```python
from build123d import *
from OCP.BRepFilletAPI import BRepFilletAPI_MakeChamfer

# Parameters (mm, degrees)
SKETCH1_W           = 76.962
SKETCH1_H           = 46.99
BOSS_EXTRUDE1_DEPTH = 20.066
SKETCH2_W           = 72.68972
SKETCH2_H           = 42.7482
CUT_EXTRUDE1_DEPTH  = 2.54
SKETCH3_W           = 69.38772
SKETCH3_H           = 39.37
CUT_EXTRUDE2_DEPTH  = 16.256
CHAMFER1_SIZE       = 2.54
SKETCH6_R           = 1.5875
BOSS_EXTRUDE2_DEPTH = 2.54
CUT_EXTRUDE5_DEPTH  = 97.402641646
FILLET1_R           = 2.54
SKETCH9_R           = 1.5875
BOSS_EXTRUDE3_DEPTH = 2.54
SKETCH12_W          = 1.27
SKETCH12_H          = 2.54
BOSS_EXTRUDE5_DEPTH = 1.27
CHAMFER4_SIZE       = 2.54
CHAMFER4_SIZE_2     = 9.479409052
SKETCH13_W          = 6.35
SKETCH13_H          = 11.176
SKETCH13_W_2        = 13.97
SKETCH13_H_2        = 6.35
CUT_EXTRUDE7_DEPTH  = 104.876082503
SKETCH14_W          = 2.54
SKETCH14_H          = 1.27
BOSS_EXTRUDE6_DEPTH = 2.54
CHAMFER5_SIZE       = 2.54000495
CHAMFER5_SIZE_2     = 9.479427523
CHAMFER6_SIZE       = 2.54


with BuildPart() as part:
    # Sketch1 → Boss-Extrude1 (new body)
    with BuildSketch(Plane(origin=(0, 0, 0), x_dir=(1, 0, 0), z_dir=(0, 1, 0))):
        with Locations((38.481, 23.495)):
            Rectangle(SKETCH1_W, SKETCH1_H)
    extrude(amount=BOSS_EXTRUDE1_DEPTH)

    # Sketch2 → Cut-Extrude1 (cut)
    with BuildSketch(Plane(origin=(0, 20.066, 0), x_dir=(1, 0, 0), z_dir=(0, 1, 0))):
        with Locations((38.481, 23.495)):
            Rectangle(SKETCH2_W, SKETCH2_H)
    extrude(amount=-CUT_EXTRUDE1_DEPTH, mode=Mode.SUBTRACT)

    # Sketch3 → Cut-Extrude2 (cut)
    with BuildSketch(Plane(origin=(0, 17.526, 0), x_dir=(1, 0, 0), z_dir=(0, 1, 0))):
        with Locations((38.481, 23.495)):
            Rectangle(SKETCH3_W, SKETCH3_H)
    extrude(amount=-CUT_EXTRUDE2_DEPTH, mode=Mode.SUBTRACT)

    # Chamfer1
    chamfer1_edges = [part.edges().sort_by_distance(p)[0] for p in [
        (0, 10.033, -46.99),
        (76.962, 10.033, -46.99),
        (76.962, 10.033, 0),
        (0, 10.033, 0),
    ]]
    chamfer(chamfer1_edges, length=CHAMFER1_SIZE)

    # Sketch6 → Boss-Extrude2 (add)
    # profile 1 of 4: a face of its own
    with BuildSketch(Plane.XZ):
        with BuildLine():
            Line((3.4925, 3.81), (3.4925, 0))
            Line((3.4925, 0), (11.7475, 0))
            Line((11.7475, 0), (11.7475, 3.81))
            ThreePointArc((11.7475, 3.81), (7.62, 7.9375), (3.4925, 3.81))
        make_face()
        with Locations(Location((7.62, 3.81, 0), (0, 0, 270))):
            Circle(SKETCH6_R, mode=Mode.SUBTRACT)
    # profile 2 of 4: a face of its own
    with BuildSketch(Plane.XZ):
        with BuildLine():
            Line((11.7475, -46.99), (11.7475, -50.8))
            ThreePointArc((11.7475, -50.8), (7.62, -54.9275), (3.4925, -50.8))
            Line((3.4925, -50.8), (3.4925, -46.99))
            Line((3.4925, -46.99), (11.7475, -46.99))
        make_face()
        with Locations(Location((7.62, -50.8, 0), (0, 0, 90))):
            Circle(SKETCH6_R, mode=Mode.SUBTRACT)
    # profile 3 of 4: a face of its own
    with BuildSketch(Plane.XZ):
        with BuildLine():
            Line((73.4695, -50.8), (73.4695, -46.99))
            Line((73.4695, -46.99), (65.2145, -46.99))
            Line((65.2145, -46.99), (65.2145, -50.8))
            ThreePointArc((65.2145, -50.8), (69.342, -54.9275), (73.4695, -50.8))
        make_face()
        with Locations(Location((69.342, -50.8, 0), (0, 0, 270))):
            Circle(SKETCH6_R, mode=Mode.SUBTRACT)
    # profile 4 of 4: a face of its own
    with BuildSketch(Plane.XZ):
        with BuildLine():
            Line((65.2145, 0), (65.2145, 3.81))
            ThreePointArc((65.2145, 3.81), (69.342, 7.9375), (73.4695, 3.81))
            Line((73.4695, 3.81), (73.4695, 0))
            Line((73.4695, 0), (65.2145, 0))
        make_face()
        with Locations(Location((69.342, 3.81, 0), (0, 0, 90))):
            Circle(SKETCH6_R, mode=Mode.SUBTRACT)
    extrude(amount=-BOSS_EXTRUDE2_DEPTH)

    # Sketch7 → Cut-Extrude5 (cut, through all)
    with BuildSketch(Plane(origin=(0, 1.27, 0), x_dir=(1, 0, 0), z_dir=(0, 1, 0))):
        Polygon((15.896309728, 40.64), (61.065690272, 40.64), (38.481, 26.492218855), align=None)
        Polygon((6.32714, 40.64), (6.32714, 6.35), (33.696415136, 23.495), align=None)
        Polygon((15.964259965, 6.392566228), (60.997740035, 6.392566228), (38.481, 20.497781145), align=None)
        Polygon((70.63486, 40.64), (70.63486, 6.35), (43.265584864, 23.495), align=None)
    extrude(amount=-CUT_EXTRUDE5_DEPTH, mode=Mode.SUBTRACT)

    # Fillet1
    fillet1_edges = [part.edges().sort_by_distance(p)[0] for p in [
        (61.065690272, 0.635, -40.64),
        (38.481, 0.635, -26.492218855),
        (15.896309728, 0.635, -40.64),
        (15.964259965, 0.635, -6.392566228),
        (38.481, 0.635, -20.497781145),
        (60.997740035, 0.635, -6.392566228),
        (43.265584864, 0.635, -23.495),
        (70.63486, 0.635, -40.64),
        (70.63486, 0.635, -6.35),
        (33.696415136, 0.635, -23.495),
        (6.32714, 0.635, -6.35),
        (6.32714, 0.635, -40.64),
    ]]
    fillet(fillet1_edges, radius=FILLET1_R)

    # Sketch9 → Boss-Extrude3 (add)
    # profile 1 of 2: a face of its own
    with BuildSketch(Plane(origin=(0, 20.066, 0), x_dir=(1, 0, 0), z_dir=(0, 1, 0))):
        with BuildLine():
            Line((-3.81, 28.575), (0, 28.575))
            Line((0, 28.575), (0, 18.415))
            Line((0, 18.415), (-3.81, 18.415))
            ThreePointArc((-3.81, 18.415), (-8.89, 23.495), (-3.81, 28.575))
        make_face()
        with Locations(Location((-3.81, 23.495, 0), (0, 0, 270))):
            Circle(SKETCH9_R, mode=Mode.SUBTRACT)
    # profile 2 of 2: a face of its own
    with BuildSketch(Plane(origin=(0, 20.066, 0), x_dir=(1, 0, 0), z_dir=(0, 1, 0))):
        with BuildLine():
            Line((76.962, 18.415), (80.772, 18.415))
            ThreePointArc((80.772, 18.415), (85.852, 23.495), (80.772, 28.575))
            Line((80.772, 28.575), (76.962, 28.575))
            Line((76.962, 28.575), (76.962, 18.415))
        make_face()
        with Locations(Location((80.772, 23.495, 0), (0, 0, 90))):
            Circle(SKETCH9_R, mode=Mode.SUBTRACT)
    extrude(amount=-BOSS_EXTRUDE3_DEPTH)

    # Sketch12 → Boss-Extrude5 (add)
    with BuildSketch(Plane(origin=(0, 2.54, 0), x_dir=(1, 0, 0), z_dir=(0, 1, 0))):
        with Locations((4.1275, -1.27)):
            Rectangle(SKETCH12_W, SKETCH12_H)
        with Locations((11.1125, -1.27)):
            Rectangle(SKETCH12_W, SKETCH12_H)
        with Locations((11.1125, 48.26)):
            Rectangle(SKETCH12_W, SKETCH12_H)
        with Locations((4.1275, 48.26)):
            Rectangle(SKETCH12_W, SKETCH12_H)
        with Locations((72.8345, 48.26)):
            Rectangle(SKETCH12_W, SKETCH12_H)
        with Locations((65.8495, 48.26)):
            Rectangle(SKETCH12_W, SKETCH12_H)
        with Locations((65.8495, -1.27)):
            Rectangle(SKETCH12_W, SKETCH12_H)
        with Locations((72.8345, -1.27)):
            Rectangle(SKETCH12_W, SKETCH12_H)
    extrude(amount=BOSS_EXTRUDE5_DEPTH)

    # Chamfer4
    chamfer4_edges_1 = [part.edges().sort_by_distance(p)[0] for p in [
        (4.1275, 3.81, -46.99),
    ]]
    chamfer4_side_1 = [part.faces().sort_by_distance(p)[0] for p in [
        (4.1275, 3.81, -47.0408),
    ]]
    chamfer4_edges_2 = [part.edges().sort_by_distance(p)[0] for p in [
        (11.1125, 3.81, -46.99),
    ]]
    chamfer4_side_2 = [part.faces().sort_by_distance(p)[0] for p in [
        (11.1125, 3.81, -47.0408),
    ]]
    chamfer4_edges_3 = [part.edges().sort_by_distance(p)[0] for p in [
        (65.8495, 3.81, -46.99),
    ]]
    chamfer4_side_3 = [part.faces().sort_by_distance(p)[0] for p in [
        (65.8495, 3.81, -47.0408),
    ]]
    chamfer4_edges_4 = [part.edges().sort_by_distance(p)[0] for p in [
        (72.8345, 3.81, -46.99),
    ]]
    chamfer4_side_4 = [part.faces().sort_by_distance(p)[0] for p in [
        (72.8345, 3.81, -47.0408),
    ]]
    chamfer4_edges_5 = [part.edges().sort_by_distance(p)[0] for p in [
        (65.8495, 3.81, 0),
    ]]
    chamfer4_side_5 = [part.faces().sort_by_distance(p)[0] for p in [
        (65.8495, 3.81, 0.0508),
    ]]
    chamfer4_edges_6 = [part.edges().sort_by_distance(p)[0] for p in [
        (72.8345, 3.81, 0),
    ]]
    chamfer4_side_6 = [part.faces().sort_by_distance(p)[0] for p in [
        (72.8345, 3.81, 0.0508),
    ]]
    chamfer4_edges_7 = [part.edges().sort_by_distance(p)[0] for p in [
        (11.1125, 3.81, 0),
    ]]
    chamfer4_side_7 = [part.faces().sort_by_distance(p)[0] for p in [
        (11.1125, 3.81, 0.0508),
    ]]
    chamfer4_edges_8 = [part.edges().sort_by_distance(p)[0] for p in [
        (4.1275, 3.81, 0),
    ]]
    chamfer4_side_8 = [part.faces().sort_by_distance(p)[0] for p in [
        (4.1275, 3.81, 0.0508),
    ]]
    chamfer4 = BRepFilletAPI_MakeChamfer(part.part.solid().wrapped)
    for e in chamfer4_edges_1:
        chamfer4.Add(CHAMFER4_SIZE - 0.0001, CHAMFER4_SIZE_2 - 0.0001, e.wrapped, chamfer4_side_1[0].wrapped)
    for e in chamfer4_edges_2:
        chamfer4.Add(CHAMFER4_SIZE - 0.0001, CHAMFER4_SIZE_2 - 0.0001, e.wrapped, chamfer4_side_2[0].wrapped)
    for e in chamfer4_edges_3:
        chamfer4.Add(CHAMFER4_SIZE - 0.0001, CHAMFER4_SIZE_2 - 0.0001, e.wrapped, chamfer4_side_3[0].wrapped)
    for e in chamfer4_edges_4:
        chamfer4.Add(CHAMFER4_SIZE - 0.0001, CHAMFER4_SIZE_2 - 0.0001, e.wrapped, chamfer4_side_4[0].wrapped)
    for e in chamfer4_edges_5:
        chamfer4.Add(CHAMFER4_SIZE - 0.0001, CHAMFER4_SIZE_2 - 0.0001, e.wrapped, chamfer4_side_5[0].wrapped)
    for e in chamfer4_edges_6:
        chamfer4.Add(CHAMFER4_SIZE - 0.0001, CHAMFER4_SIZE_2 - 0.0001, e.wrapped, chamfer4_side_6[0].wrapped)
    for e in chamfer4_edges_7:
        chamfer4.Add(CHAMFER4_SIZE - 0.0001, CHAMFER4_SIZE_2 - 0.0001, e.wrapped, chamfer4_side_7[0].wrapped)
    for e in chamfer4_edges_8:
        chamfer4.Add(CHAMFER4_SIZE - 0.0001, CHAMFER4_SIZE_2 - 0.0001, e.wrapped, chamfer4_side_8[0].wrapped)
    add(Compound.cast(chamfer4.Shape()), mode=Mode.REPLACE)  # a hair under: the kernel refuses the full size

    # Sketch13 → Cut-Extrude7 (cut, through all)
    with BuildSketch(Plane.ZY):
        with Locations((-23.495, 6.858)):
            Rectangle(SKETCH13_W, SKETCH13_H)
        with Locations((-36.195, 4.445)):
            Rectangle(SKETCH13_W_2, SKETCH13_H_2)
        with Locations((-10.795, 4.445)):
            Rectangle(SKETCH13_W_2, SKETCH13_H_2)
    extrude(amount=-CUT_EXTRUDE7_DEPTH, mode=Mode.SUBTRACT)

    # Sketch14 → Boss-Extrude6 (add)
    with BuildSketch(Plane.XZ.offset(-17.526)):
        with Locations((-1.27, -19.05)):
            Rectangle(SKETCH14_W, SKETCH14_H)
        with Locations((-1.27, -27.94)):
            Rectangle(SKETCH14_W, SKETCH14_H)
        with Locations((78.232, -27.94)):
            Rectangle(SKETCH14_W, SKETCH14_H)
        with Locations((78.232, -19.05)):
            Rectangle(SKETCH14_W, SKETCH14_H)
    extrude(amount=BOSS_EXTRUDE6_DEPTH)

    # Chamfer5
    chamfer5_edges_1 = [part.edges().sort_by_distance(p)[0] for p in [
        (76.962, 14.986, -19.05),
    ]]
    chamfer5_side_1 = [part.faces().sort_by_distance(p)[0] for p in [
        (77.012800099, 14.986, -19.05),
    ]]
    chamfer5_edges_2 = [part.edges().sort_by_distance(p)[0] for p in [
        (76.962, 14.986, -27.94),
    ]]
    chamfer5_side_2 = [part.faces().sort_by_distance(p)[0] for p in [
        (77.012800099, 14.986, -27.94),
    ]]
    chamfer5_edges_3 = [part.edges().sort_by_distance(p)[0] for p in [
        (0, 14.986, -27.94),
    ]]
    chamfer5_side_3 = [part.faces().sort_by_distance(p)[0] for p in [
        (-0.050800099, 14.986, -27.94),
    ]]
    chamfer5_edges_4 = [part.edges().sort_by_distance(p)[0] for p in [
        (0, 14.986, -19.05),
    ]]
    chamfer5_side_4 = [part.faces().sort_by_distance(p)[0] for p in [
        (-0.050800099, 14.986, -19.05),
    ]]
    chamfer5 = BRepFilletAPI_MakeChamfer(part.part.solid().wrapped)
    for e in chamfer5_edges_1:
        chamfer5.Add(CHAMFER5_SIZE - 0.0001, CHAMFER5_SIZE_2 - 0.0001, e.wrapped, chamfer5_side_1[0].wrapped)
    for e in chamfer5_edges_2:
        chamfer5.Add(CHAMFER5_SIZE - 0.0001, CHAMFER5_SIZE_2 - 0.0001, e.wrapped, chamfer5_side_2[0].wrapped)
    for e in chamfer5_edges_3:
        chamfer5.Add(CHAMFER5_SIZE - 0.0001, CHAMFER5_SIZE_2 - 0.0001, e.wrapped, chamfer5_side_3[0].wrapped)
    for e in chamfer5_edges_4:
        chamfer5.Add(CHAMFER5_SIZE - 0.0001, CHAMFER5_SIZE_2 - 0.0001, e.wrapped, chamfer5_side_4[0].wrapped)
    add(Compound.cast(chamfer5.Shape()), mode=Mode.REPLACE)  # a hair under: the kernel refuses the full size

    # Chamfer6
    chamfer6_edges = [part.edges().sort_by_distance(p)[0] for p in [
        (75.06843, 7.62, -43.18),
        (1.89357, 7.62, -43.18),
        (75.06843, 7.62, -29.21),
        (1.89357, 7.62, -29.21),
        (75.06843, 7.62, -17.78),
        (1.89357, 7.62, -17.78),
        (75.06843, 7.62, -3.81),
        (1.89357, 7.62, -3.81),
    ]]
    chamfer(chamfer6_edges, length=CHAMFER6_SIZE)


solid = part.part
```
Can you work these out from the model? Positions are in its coordinate system, mm. A direction names the side the tool comes from. Coordinates: 2 decimals unless noted, no trailing zeros. Write each loop counter-clockwise with the first axis right and the second up, starting at its lowest first coordinate (ties: lowest second). Pieces come first, ordered by that corner, then holes. Notation, with made-up numbers: M 28,10 L 35,10 A20 cw 35,44 Z; hole C 37.25,-31 d4. An arc over 180 degrees is marked long. Write item = value, one per line. Start each with the question number.
Q1. If we section it at C-C, the plane z = -1: Write out the boundary of the cut face in (x, y), then the cut area to 3 significant figures.
Q2. If we section it at A-A, the plane x = 7.62: Write out the boundary of the cut face in (y, z).
Q3. I'm going to push flat-ended pins straight in: pin 1 (1.3 mm diameter, centred on x = 77.5, y = 13, fed in from +Z); pin 2 (5 mm diameter, centred on y = 5, z = -4.5, fed in from +X); pin 3 (3 mm diameter, centred on y = 10, z = -48, fed in from -X). Where does each tip first touch, or does it pass through?
Q4. Thinking about a two-plate mould opening in X: for faces 5 (the face through (72.83, 8.62, 1.25)), 6 (the face through (-1.252, 10.18, -19.059)), 7 (the face through (73.175, 13, -23)), which applies, released by +X, released by -X, zero draft, split by the parting line, or undercut?
Q5. On a 3-axis mill with a long thin cutter (end or side, diameter ignored), from which of +Z, -Z, +X, -X, +Y, -Y can I reach the whole of each face in a straight line? I mean faces 1 (the face through (4.762, 7, -48)), 2 (the face through (10.478, 7, 1)), 3 (the face through (69.292, 0.626, -38.292)), 4 (the face through (75, 3, -29.21)). Say none if no direction works.
Q6. If I drill on L1, parallel to Z at x = 6, y = 7.5; L2, parallel to X at y = 11.5, z = -32.5; L3, parallel to Y at x = 33.5, z = -22, over which ranges is the centre line in solid material (lowest first)? Write a range as [from, to].
Q7. If we section it at B-B, the plane x = 35: Write out the boundary of the cut face in (y, z).
Check sheet entries:
q1.outline = M 1.54,0 L 75.42,0 L 75.42,20.07 L 1.54,20.07 Z
q1.area = 1,480 mm²
q2.outline = M 0,-54.93 L 2.54,-54.93 L 2.54,-52.39 L 0,-52.39 Z; M 0,-49.21 L 2.54,-49.21 L 2.54,-46.99 L 20.07,-46.99 L 20.07,-44.87 L 17.53,-44.87 L 17.53,-43.18 L 1.27,-43.18 L 1.27,-38.26 L 0,-38.26 Z; M 0,-8.73 L 1.27,-8.73 L 1.27,-3.81 L 17.53,-3.81 L 17.53,-2.12 L 20.07,-2.12 L 20.07,0 L 2.54,0 L 2.54,2.22 L 0,2.22 Z; M 0,5.4 L 2.54,5.4 L 2.54,7.94 L 0,7.94 Z
q3.pin_1 = -2.43
q3.pin_2 = 76.96
q3.pin_3 = 2.05
q4.face_5 = zero draft
q4.face_6 = released by -X
q4.face_7 = undercut
q5.face_1 = -Z, +Y
q5.face_2 = +Z, +Y
q5.face_3 = +Y, -Y
q5.face_4 = +X, -X
q6.L1 = [-46.99, -43.18], [-3.81, 0]
q6.L2 = [0, 3.79], [73.17, 76.96]
q6.L3 = [0, 1.27]
q7.outline = M 0,-46.99 L 20.07,-46.99 L 20.07,-44.87 L 17.53,-44.87 L 17.53,-43.18 L 1.27,-43.18 L 1.27,-40.64 L 0,-40.64 Z; M 0,-28.67 L 1.27,-28.67 L 1.27,-18.32 L 0,-18.32 Z; M 0,-6.39 L 1.27,-6.39 L 1.27,-3.81 L 17.53,-3.81 L 17.53,-2.12 L 20.07,-2.12 L 20.07,0 L 0,0 Z
